Geometry check sheet. Reference: the model listing, model coordinates, mm. Face numbers are marked on the shaded views. Give positions to 0.01 mm unless a question says otherwise; leave off trailing zeros. Order: outer loops, then holes, each group sorted by start corner. A loop starts at its lowest first (then second) coordinate and runs counter-clockwise, first axis right, second up. Notation, with made-up numbers: M 89.5,81 L 144.5,81 A29 ccw 144.5,111 Z; hole C 9.25,51 d10. An arc over 180 degrees is marked long. Put each result on its own line as item: value. Start each with the question number.
Q1. Material ranges on L1, parallel to Y at x = 122, z = -0.75; L2, parallel to Z at x = 83, y = -19; L3, parallel to Z at x = -200.5, y = -8.5, recorded low to high.
Q2. Go/stop test with flat-tipped pins: pin 1 (1 mm diameter, centred on x = 73.5, y = -16.5, fed in from +Z); pin 2 (5 mm diameter, centred on x = 105.5, z = 2.5, fed in from -Y); pin 3 (1 mm diameter, centred on x = -123.5, y = -21, fed in from -Z). Record where each tip stops, or that it passes through.
Q3. Section check A-A on x = -103. Record the cut outline in (y, z), then the cut area to 3 significant figures.
Q4. Mould release check, pull along Y, two halves, no side actions. Record for the marked faces 1 and 2: +Y half, -Y half, draft (parallel to the pull), parting line (faces both ways), or undercut.
Q5. Section check B-B on y = -5.5. Record the cut outline in (x, z).
```python
from build123d import *

# Parameters (mm, degrees)
BASE_FLANGE1_START = -229.4001
BASE_FLANGE1_DEPTH = 458.8002
SKETCH3_R          = 2.1082
CUT_EXTRUDE1_DEPTH = 232.388150944
CUT_EXTRUDE2_DEPTH = 1.016


# Read off the part's stored shape, not the designer's step: Base-Flange1
with BuildPart() as part:
    # Base-Flange1 outline → Base-Flange1 (new body)
    with BuildSketch(Plane(origin=(0, 0, 0), x_dir=(0, 0, -1), z_dir=(1, 0, 0)).offset(BASE_FLANGE1_START)):
        with BuildLine():
            ThreePointArc((-13.368341311, -20.466361656), (-13.309368584, -21.067196635), (-12.979624418, -21.572913195))
            Line((-12.979624418, -21.572913195), (-7.031153987, -27.148026486))
            Line((-7.031153987, -27.148026486), (-6.336374453, -26.406718588))
            Line((-6.336374453, -26.406718588), (-12.284844884, -20.831605297))
            ThreePointArc((-12.284844884, -20.831605297), (-12.350793717, -20.730461985), (-12.362588262, -20.610294989))
            Line((-12.362588262, -20.610294989), (-9.589648793, -1.234016667))
            ThreePointArc((-9.589648793, -1.234016667), (-9.504607996, -1.078094077), (-9.33821053, -1.016))
            Line((-9.33821053, -1.016), (5.5626, -1.016))
            Line((5.5626, -1.016), (5.5626, 0))
            Line((5.5626, 0), (-9.33821053, 0))
            ThreePointArc((-9.33821053, 0), (-10.17019786, -0.310470384), (-10.595401842, -1.090083333))
            Line((-10.595401842, -1.090083333), (-13.368341311, -20.466361656))
        make_face()
    extrude(amount=BASE_FLANGE1_DEPTH)

    # Sketch3 → Cut-Extrude1 (cut, through all)
    with BuildSketch(Plane(origin=(0, 0, 0), x_dir=(1, 0, 0), z_dir=(0, 1, 0))):
        with Locations(Location((-38.1, 0, 0), (0, 0, 270))):
            Circle(SKETCH3_R)
        with Locations(Location((-114.3, 0, 0), (0, 0, 270))):
            Circle(SKETCH3_R)
        with Locations(Location((-190.5, 0, 0), (0, 0, 270))):
            Circle(SKETCH3_R)
        with Locations(Location((190.5, 0, 0), (0, 0, 270))):
            Circle(SKETCH3_R)
        with Locations(Location((114.3, 0, 0), (0, 0, 270))):
            Circle(SKETCH3_R)
        with Locations(Location((38.1, 0, 0), (0, 0, 270))):
            Circle(SKETCH3_R)
    extrude(amount=-CUT_EXTRUDE1_DEPTH, mode=Mode.SUBTRACT)

    # Sketch4 → Cut-Extrude2 (cut)
    with BuildSketch(Plane(origin=(0, 0, 0), x_dir=(1, 0, 0), z_dir=(0, 1, 0))):
        Polygon((-215.810037107, 6.452662893), (-235.374711333, -13.112011333), (-235.374711333, 6.452662893), align=None)
        Polygon((235.374711333, 6.452662893), (215.810037107, 6.452662893), (235.374711333, -13.112011333), align=None)
    extrude(amount=-CUT_EXTRUDE2_DEPTH, mode=Mode.SUBTRACT)


solid = part.part
```
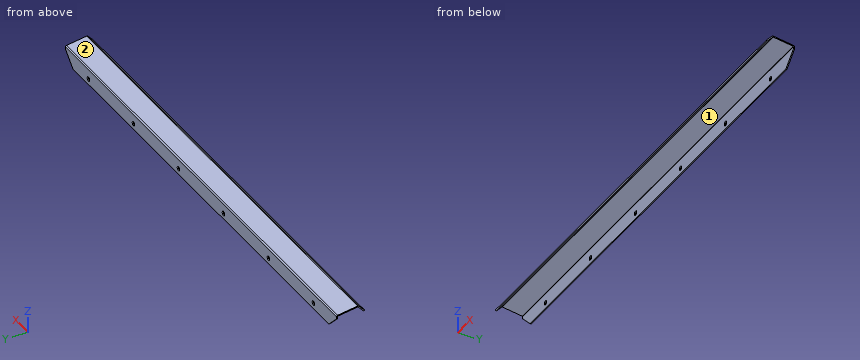
Results found:
1. L1: y = -1.02 to 0
1. L2: z = 12.13 to 13.16
1. L3: z = 10.63 to 11.66
2. pin 1: stops at z = 12.87
2. pin 2: stops at y = -1.02
2. pin 3: stops at z = 11.57
3. outline: M -27.15,7.03 L -26.41,6.34 L -20.83,12.28 A0.25 cw -20.61,12.36 L -1.23,9.59 A0.25 cw -1.02,9.34 L -1.02,-5.56 L 0,-5.56 L 0,9.34 A1.27 ccw -1.09,10.6 L -20.47,13.37 A1.27 ccw -21.57,12.98 Z
3. area: 45.2 mm^2
4. face 1: undercut
4. face 2: +Y half
5. outline: M -229.4,10.2 L 229.4,10.2 L 229.4,11.23 L -229.4,11.23 Z
